The figure shows three views and two pictorial views of one solid part (mm, origin at its lowest corner). Answer the questions. A direction names the side the tool comes from. Coordinates: 2 decimals unless noted, no trailing zeros. Loops run counter-clockwise (first coordinate to the right, second up) from the corner with the lowest first, then second, coordinate; pieces in that order, holes last. Notation, with made-up numbers: M 67,56 L 102,56 A10 ccw 102,65 Z; hole C 6.25,48.25 d3. An arc over 180 degrees is marked long. Write each question's results on one line, items separated by ' | '.
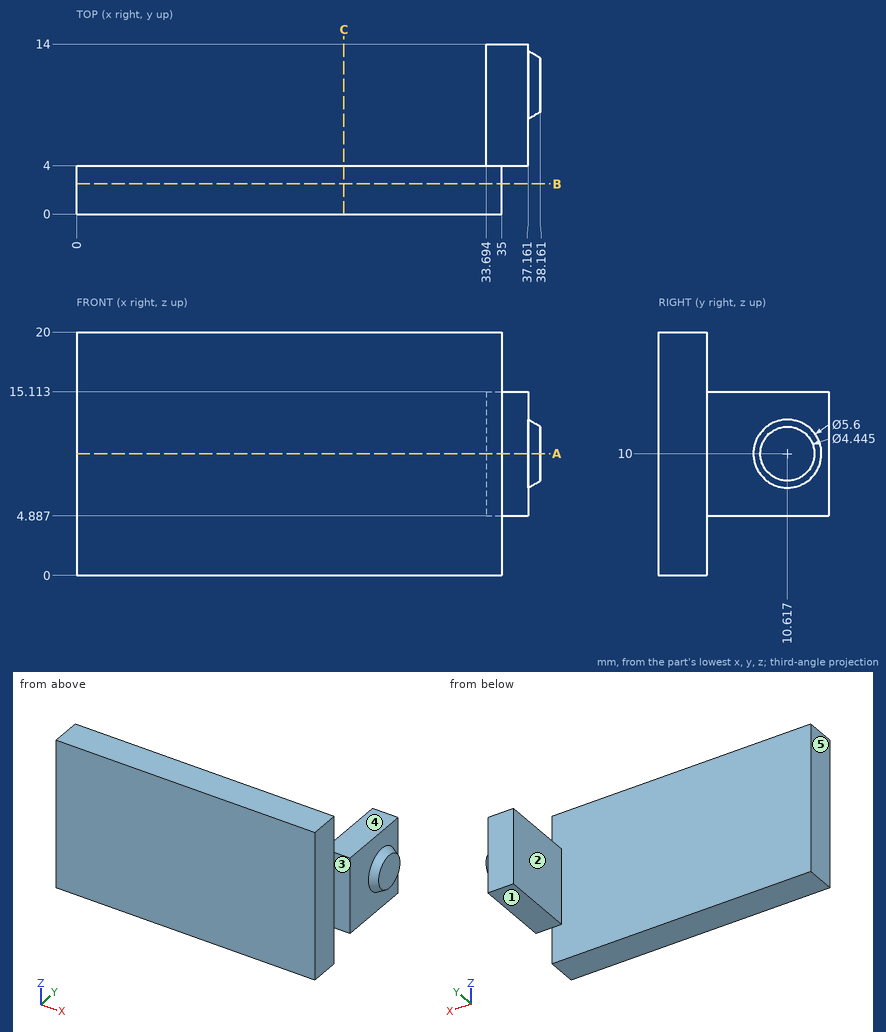
1) Find section B-B, the plane y = 2.5. Give the vertices of the cut face in (x, z), and give its area (3 significant figures).
Check result:
outline: M 0,0 L 35,0 L 35,20 L 0,20 Z | area: 700 mm^2
2) Which of the six approach directions +Z, -Z, +X, -X, +Y, -Y give full straight-line access (tool end or side, diameter ignored) to the marked faces 1, 2, 3, 4 and 5?
Check result:
face 1: -Z, +X, -X, +Y | face 2: +Z, -Z, -X, +Y | face 3: +Z, -Z, +X, -Y | face 4: +Z, +X, -X, +Y | face 5: +Z, -Z, -X, +Y, -Y
3) Straight lines are drawn through the part: probe 1 along Y at (x, z) = (12, 15.25); probe 2 along X at (y, z) = (7, 13.75) (1 decimal); probe 3 along X at (y, z) = (12.25, 9) (1 decimal). For each, find the intervals that lie inside material, in ascending order. Write a range as [from, to].
Check result:
probe 1: [0, 4] | probe 2: [33.7, 37.2] | probe 3: [33.7, 38.2]
4) Find section A-A, the plane z = 10. Give the vertices of the cut face in (x, y) (1 decimal).
Check result:
outline: M 0,0 L 35,0 L 35,4 L 37.2,4 L 37.2,7.8 L 38.2,8.4 L 38.2,12.8 L 37.2,13.4 L 37.2,14 L 33.7,14 L 33.7,4 L 0,4 Z
5) Find section C-C, the plane x = 22. Give the vertices of the cut face in (y, z).
Check result:
outline: M 0,0 L 4,0 L 4,20 L 0,20 Z
6) Given pin 1 Ø1 at (x, y) = (35, 9) entering from +Z; pin 2 Ø8 at (x, y) = (20.5, 11.5) entering from +Z; pin 3 Ø5 at (x, z) = (27.5, 8.5) entering from -Y; pin 4 Ø2 at (y, z) = (2, 11) entering from +X, each flat-ended and moving along its own axis, determine where each tip first touches the part or whether it passes through.
Check result:
pin 1: z = 15.11 | pin 2: through | pin 3: y = 0 | pin 4: x = 35
